For this review, take the finished solid that the model builds, in its own axes (mm). A direction names the side the tool comes from. Coordinates: 2 decimals unless noted, no trailing zeros. Write each loop counter-clockwise with the first axis right and the second up, starting at its lowest first coordinate (ties: lowest second). Pieces come first, ordered by that corner, then holes. Notation, with made-up numbers: M 55,22.25 L 112,22.25 A27 ccw 112,42.25 Z; hole C 33.5,27.25 d5. An arc over 180 degrees is marked long. Return JSON: item names as keys, results as strings.
```python
from build123d import *

# Parameters (mm, degrees)
F1_DEPTH = 150
F2_W     = 16
F2_H     = 130
F3_DEPTH = 170
F5_DEPTH = 16
F6_R     = 6
F7_DEPTH = 15
F8_R     = 6
F9_DEPTH = 20


with BuildPart() as f1:
    # F0 (on Front) → F1 (new body)
    with BuildSketch(Plane.XZ):
        Polygon((-95.860116, -70.643179), (-75.860116, -70.643179), (-75.860116, 79.356821), (104.139884, 79.356821), (104.139884, 94.356821), (-95.860116, 94.356821), align=None)
    extrude(amount=F1_DEPTH)

    # F2 (on face) → F3 (join)
    with BuildSketch(Plane.YZ.offset(-75.860116)):
        with Locations((-75, 14.356821)):
            Rectangle(F2_W, F2_H)
    extrude(amount=F3_DEPTH)

    # F4 (on face) → F5 (cut)
    with BuildSketch(Plane.XZ.offset(83)):
        with BuildLine():
            ThreePointArc((-44.365328, -49.667342), (-45.934238, -50.394048), (-47.645235, -50.643179))
            Line((-47.645235, -50.643179), (94.139884, -50.643179))
            Line((94.139884, -50.643179), (94.139884, 48.873568))
            ThreePointArc((94.139884, 48.873568), (92.330723, 41.732018), (87.339651, 36.313161))
            Line((87.339651, 36.313161), (-44.365328, -49.667342))
        make_face()
    extrude(amount=-F5_DEPTH, mode=Mode.SUBTRACT)

    # F6 (on face) → F7 (cut)
    with BuildSketch(Plane.XY.offset(94.356821)):
        with Locations((-25.860116, -25)):
            Circle(F6_R)
        with Locations((24.139884, -25)):
            Circle(F6_R)
        with Locations((74.139884, -25)):
            Circle(F6_R)
        with Locations((74.139884, -125)):
            Circle(F6_R)
        with Locations((24.139884, -125)):
            Circle(F6_R)
        with Locations((-25.860116, -125)):
            Circle(F6_R)
    extrude(amount=-F7_DEPTH, mode=Mode.SUBTRACT)

    # F8 (on face) → F9 (cut)
    with BuildSketch(Plane(origin=(-95.860116, 0, 0), x_dir=(0, -1, 0), z_dir=(-1, 0, 0))):
        with Locations((125, 29.356821)):
            Circle(F8_R)
        with Locations((125, -45.643179)):
            Circle(F8_R)
        with Locations((25, -45.643179)):
            Circle(F8_R)
        with Locations((25, 29.356821)):
            Circle(F8_R)
    extrude(amount=-F9_DEPTH, mode=Mode.SUBTRACT)


solid = f1.part
```
1. Wall thickness on L1, parallel to Z at x = -84, y = -125; L2, parallel to Z at x = -23, y = -47; L3, parallel to Y at x = -15, z = 41: over which ranges is each line inside the solid? List them lowest first. Write a range as from..to.
Checks:
{"L1": "-70.64..-51.64, -39.64..23.36, 35.36..94.36", "L2": "79.36..94.36", "L3": "-83..-67"}
2. For faces 4 (the face through (-62, -75, -50.643)), 5 (the face through (-11, -67, 28)), 6 (the face through (6, -74, 94.357)), list the 3-axis set-ups (+Z, -Z, +X, -X, +Y, -Y) from which the entire face can be reached by the end or side of a thin tool; tool diameter is ignored.
Checks:
{"face 4": "-Z, +X, +Y, -Y", "face 5": "-Z, +X, +Y", "face 6": "+Z, +X, -X, +Y, -Y"}
3. We need section C-C (x = -52). State the section outline as (y, z) points.
Checks:
{"outline": "M -150,79.36 L -83,79.36 L -83,-50.64 L -67,-50.64 L -67,79.36 L 0,79.36 L 0,94.36 L -150,94.36 Z"}
4. We need section B-B (z = 73). State the section outline as (x, y) points, plus the area to 3 significant figures.
Checks:
{"outline": "M -95.86,-150 L -75.86,-150 L -75.86,-83 L 94.14,-83 L 94.14,-67 L -75.86,-67 L -75.86,0 L -95.86,0 Z", "area": "5,720 mm2"}
5. We need section D-D (z = -59). State the section outline as (x, y) points.
Checks:
{"outline": "M -95.86,-150 L -75.86,-150 L -75.86,0 L -95.86,0 Z"}
6. We need section A-A (y = -25). State the section outline as (x, z) points, plus the area to 3 significant figures.
Checks:
{"outline": "M -95.86,-70.64 L -75.86,-70.64 L -75.86,-51.64 L -95.86,-51.64 Z; M -95.86,-39.64 L -75.86,-39.64 L -75.86,23.36 L -95.86,23.36 Z; M -95.86,35.36 L -75.86,35.36 L -75.86,79.36 L -31.86,79.36 L -31.86,94.36 L -95.86,94.36 Z; M -19.86,79.36 L 18.14,79.36 L 18.14,94.36 L -19.86,94.36 Z; M 30.14,79.36 L 68.14,79.36 L 68.14,94.36 L 30.14,94.36 Z; M 80.14,79.36 L 104.14,79.36 L 104.14,94.36 L 80.14,94.36 Z", "area": "4,980 mm2"}
7. Draft analysis for pull direction Z (two halves, no side actions). For faces 1 (the face through (-75.86, -91, 3)), 2 (the face through (-86, -119.006, -45.379)), 3 (the face through (92.38, -75.11, 41.82)), state which applies: +Z half, -Z half, draft (parallel to the pull), parting line (faces both ways), or undercut.
Checks:
{"face 1": "draft", "face 2": "undercut", "face 3": "-Z half"}
8. Clearance check with flat-ended pins moving along their axes: pin 1 Ø1 at (x, z) = (64, 18.5) entering from -Y; pin 2 Ø19 at (y, z) = (-25, -45.64) entering from +X; pin 3 Ø5 at (y, z) = (-78, 61) entering from +X; pin 4 Ø15.5 at (x, y) = (74.14, -25) entering from +Z. State where each tip first meets the part, or that it passes through.
Checks:
{"pin 1": "through", "pin 2": "x = -75.86", "pin 3": "x = 94.14", "pin 4": "z = 94.36"}
